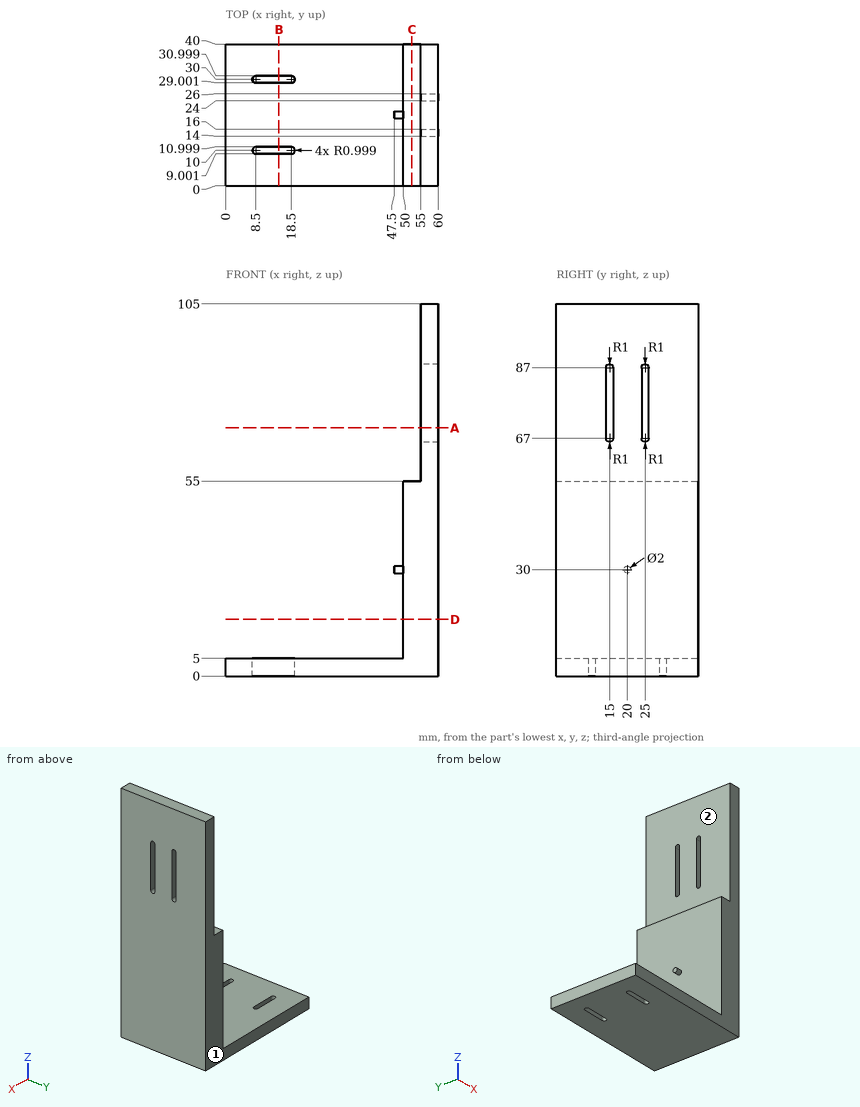
Geometry check sheet. Reference: drawing and pictorial views, mm from the part's lowest x, y, z. A direction names the side the tool comes from. Coordinates: 2 decimals unless noted, no trailing zeros. Loops run counter-clockwise (first coordinate to the right, second up) from the corner with the lowest first, then second, coordinate; pieces in that order, holes last. Notation, with made-up numbers: (85, 38) -> (141, 38) arc R25 ccw to (141, 65) -> close; hole circle Ø3 at (-12, 12.5). An arc over 180 degrees is marked (long way). Put each result on its own line as item: value.
1) Cross-section at C-C on x = 52.5. Record the boundary of the cut face in (y, z), plus the area to 3 significant figures.
Result set:
outline: (0, 0) -> (40, 0) -> (40, 55) -> (0, 55) -> close
area: 2,200 mm^2
2) Tool access check on the marked faces 1 and 2. Record the directions out of +Z, -Z, +X, -X, +Y, -Y that give a thin tool (end or side, any length) a straight path to the whole face; none if there is none.
Result set:
face 1: +Z, -Z, +X, -X, +Y
face 2: +Z, -X, +Y, -Y
3) Cross-section at D-D on z = 16. Record the boundary of the cut face in (x, y), plus the area to 3 significant figures.
Result set:
outline: (50, 0) -> (60, 0) -> (60, 40) -> (50, 40) -> close
area: 400 mm^2
4) Gauge pin test, flat ends, axial feed: pin 1 Ø2 at (y, z) = (9.5, 93.5) entering from -X; pin 2 Ø12 at (y, z) = (28, 35.5) entering from -X; pin 3 Ø3 at (x, y) = (31, 18) entering from +Z. Record the tip position at first contact, or that the pin passes through.
Result set:
pin 1: stops at x = 55
pin 2: stops at x = 50
pin 3: stops at z = 5
5) Cross-section at B-B on x = 15. Record the boundary of the cut face in (y, z).
Result set:
outline: (0, 0) -> (9, 0) -> (9, 5) -> (0, 5) -> close; (11, 0) -> (29, 0) -> (29, 5) -> (11, 5) -> close; (31, 0) -> (40, 0) -> (40, 5) -> (31, 5) -> close
6) Cross-section at A-A on z = 70. Record the boundary of the cut face in (x, y), plus the area to 3 significant figures.
Result set:
outline: (55, 0) -> (60, 0) -> (60, 14) -> (55, 14) -> close; (55, 16) -> (60, 16) -> (60, 24) -> (55, 24) -> close; (55, 26) -> (60, 26) -> (60, 40) -> (55, 40) -> close
area: 180 mm^2
7) Thickness scan on line 1 (X direction, y = 5.5, z = 18.5); line 2 (Z direction, x = 12, y = 13); line 3 (X direction, y = 18.5, z = 72). Record the ranges inside material, lowest first.
Result set:
line 1: x = 50 to 60
line 2: z = 0 to 5
line 3: x = 55 to 60
